```python
from build123d import *
from OCP.BRepFilletAPI import BRepFilletAPI_MakeFillet

# Parameters (mm, degrees)
SKETCH1_W                 = 28
SKETCH1_H                 = 28
BOSS_EXTRUDE1_DEPTH       = 66
SHELL1_T                  = -2
SHELL1_THICKNESS_2_FACE_W = 24
SHELL1_THICKNESS_2_FACE_H = 26
SHELL1_THICKNESS_2_DEPTH  = 1
SKETCH2_R                 = 2.5
SKETCH2_R_2               = 1.425
CUT_EXTRUDE4_DEPTH        = 2
SKETCH5_W                 = 14
SKETCH5_H                 = 5
CUT_EXTRUDE6_DEPTH        = 10
SKETCH6_R                 = 7
SKETCH6_R_2               = 1.1
CUT_EXTRUDE8_DEPTH        = 10
FILLET1_R                 = 0.5
BOSS_EXTRUDE2_START       = 8
BOSS_EXTRUDE2_DEPTH       = 32
SKETCH16_W                = 4
SKETCH16_H                = 2
BOSS_EXTRUDE9_DEPTH       = 1.5
SKETCH17_W                = 2.65
SKETCH17_H                = 2.3
CUT_EXTRUDE9_DEPTH        = 3
FILLET3_R                 = 1
FILLET3_R_2               = 0.5
CUT_EXTRUDE10_REACH       = 71.226
SKETCH18_W                = 14
SKETCH18_H                = 14


with BuildPart() as part:
    # Sketch1 → Boss-Extrude1 (new body)
    with BuildSketch(Plane.XY):
        Rectangle(SKETCH1_W, SKETCH1_H)
    extrude(amount=BOSS_EXTRUDE1_DEPTH)

    # Shell1
    shell1_openings = [part.faces().sort_by_distance(p)[0] for p in [
        (0, -14, 33),
    ]]
    offset(amount=SHELL1_T, openings=shell1_openings, kind=Kind.INTERSECTION)

    # Shell1 thickness 2 face (on inner face of the shell) → Shell1 thickness 2 (cut)
    with BuildSketch(Plane(origin=(0, -1, 64), x_dir=(1, 0, 0), z_dir=(0, 0, 1))):
        Rectangle(SHELL1_THICKNESS_2_FACE_W, SHELL1_THICKNESS_2_FACE_H)
    extrude(amount=SHELL1_THICKNESS_2_DEPTH, mode=Mode.SUBTRACT)

    # Sketch2 → Cut-Extrude4 (cut)
    with BuildSketch(Plane.XY):
        Circle(SKETCH2_R)
        with Locations((8.25, 0)):
            Circle(SKETCH2_R_2)
        with Locations((0, -8.25)):
            Circle(SKETCH2_R_2)
        with Locations((-8.25, 0)):
            Circle(SKETCH2_R_2)
        with Locations((0, 8.25)):
            Circle(SKETCH2_R_2)
    extrude(amount=CUT_EXTRUDE4_DEPTH, mode=Mode.SUBTRACT)

    # Sketch5 → Cut-Extrude6 (cut)
    with BuildSketch(Plane(origin=(0, 14, 0), x_dir=(1, 0, 0), z_dir=(0, 1, 0))):
        with Locations((0, -7.5)):
            Rectangle(SKETCH5_W, SKETCH5_H)
    extrude(amount=-CUT_EXTRUDE6_DEPTH, mode=Mode.SUBTRACT)

    # Sketch6 → Cut-Extrude8 (cut)
    with BuildSketch(Plane.XY.offset(66)):
        Circle(SKETCH6_R)
        with Locations((0, 9)):
            Circle(SKETCH6_R_2)
        with Locations((9, 0)):
            Circle(SKETCH6_R_2)
        with Locations((0, -9)):
            Circle(SKETCH6_R_2)
        with Locations((-9, 0)):
            Circle(SKETCH6_R_2)
    extrude(amount=-CUT_EXTRUDE8_DEPTH, mode=Mode.SUBTRACT)

    # Fillet1
    fillet1_edges = [part.edges().sort_by_distance(p)[0] for p in [
        (-7, 13, 5),
        (7, 13, 5),
        (7, 13, 10),
        (-7, 13, 10),
    ]]
    fillet(fillet1_edges, radius=FILLET1_R)

    # Sketch9 → Boss-Extrude2 (add)
    with BuildSketch(Plane.XY.offset(2).offset(BOSS_EXTRUDE2_START)):
        with BuildLine():
            ThreePointArc((6.82202316, 7.65), (9.353829093, 4.191465293), (10.25, 0))
            Line((10.25, 0), (12, 0))
            Line((12, 0), (12, 12))
            Line((12, 12), (-12, 12))
            Line((-12, 12), (-12, 0))
            Line((-12, 0), (-10.25, 0))
            ThreePointArc((-10.25, 0), (-9.353829093, 4.191465293), (-6.82202316, 7.65))
            ThreePointArc((-6.82202316, 7.65), (0, 10.25), (6.82202316, 7.65))
        make_face()
        with BuildLine():
            Line((-6.82202316, 7.65), (-1.292526595, 7.65))
            ThreePointArc((-1.292526595, 7.65), (-0.307225163, 9.641487585), (1.425, 8.25))
            ThreePointArc((1.425, 8.25), (1.391487585, 7.942774837), (1.292526595, 7.65))
            Line((1.292526595, 7.65), (6.82202316, 7.65))
            ThreePointArc((6.82202316, 7.65), (0, 10.25), (-6.82202316, 7.65))
        make_face()
        with BuildLine():
            Line((-1.292526595, 7.65), (0, 7.65))
            Line((0, 7.65), (1.292526595, 7.65))
            ThreePointArc((1.292526595, 7.65), (1.391487585, 7.942774837), (1.425, 8.25))
            ThreePointArc((1.425, 8.25), (-0.307225163, 9.641487585), (-1.292526595, 7.65))
        make_face()
    extrude(amount=BOSS_EXTRUDE2_DEPTH)

    # Sketch16 → Boss-Extrude9 (add)
    with BuildSketch(Plane.XZ.offset(14)):
        with Locations((-2, 1)):
            Rectangle(SKETCH16_W, SKETCH16_H)
        with Locations((2, 1)):
            Rectangle(SKETCH16_W, SKETCH16_H)
    extrude(amount=BOSS_EXTRUDE9_DEPTH)

    # Sketch17 → Cut-Extrude9 (cut)
    with BuildSketch(Plane.XY.offset(2)):
        with Locations((1.325, -12.85)):
            Rectangle(SKETCH17_W, SKETCH17_H)
        with Locations((-1.325, -12.85)):
            Rectangle(SKETCH17_W, SKETCH17_H)
    extrude(amount=-CUT_EXTRUDE9_DEPTH, mode=Mode.SUBTRACT)

    # Fillet3
    fillet3_edges_1 = [part.edges().sort_by_distance(p)[0] for p in [
        (-4, -15.5, 1),
        (4, -15.5, 1),
    ]]
    fillet3_edges_2 = [part.edges().sort_by_distance(p)[0] for p in [
        (4, -14, 1),
        (-4, -14, 1),
    ]]
    fillet3 = BRepFilletAPI_MakeFillet(part.part.solid().wrapped)
    for e in fillet3_edges_1:
        fillet3.Add(FILLET3_R - 0.0001, e.wrapped)
    for e in fillet3_edges_2:
        fillet3.Add(FILLET3_R_2 - 0.0001, e.wrapped)
    add(Compound.cast(fillet3.Shape()), mode=Mode.REPLACE)  # a hair under: the kernel refuses the full size

    # Sketch18 → Cut-Extrude10 (cut, up to next)
    with BuildSketch(Plane.XY.offset(66), mode=Mode.PRIVATE) as cut_extrude10_sk1:
        with Locations((0, -7)):
            Rectangle(SKETCH18_W, SKETCH18_H)
    cut_extrude10_tool1 = extrude(cut_extrude10_sk1.sketch, amount=-CUT_EXTRUDE10_REACH, mode=Mode.PRIVATE) & part.part
    add(cut_extrude10_tool1.solids().sort_by_distance((0, -7, 66))[0], mode=Mode.SUBTRACT)


solid = part.part
```
CAD build for the part. Positions are in the model's coordinates, mm. A direction names the side the tool comes from. Round coordinates to 2 decimals unless told otherwise and drop trailing zeros. Order: outer loops, then holes, each group sorted by start corner. A loop starts at its lowest first (then second) coordinate and runs counter-clockwise, first axis right, second up. Notation, with made-up numbers: (-38, 89) -> (-10, 89) arc R22 ccw to (-10, 102) -> close; hole circle Ø6 at (-4, 44.25). An arc over 180 degrees is marked (long way). One line per question, with ' | ' between items.
Q1. Slice it at A-A (x = 0). Give the number of separate pieces and of enclosed holes in the cut face, then the cut area to 3 significant figures.
Completed:
separate pieces: 7 | enclosed holes: 0 | area: 293 mm^2
Q2. Drop flat-ended pins along their axis: pin 1 (1.5 mm diameter, centred on x = 5, y = -6, fed in from +Z); pin 2 (10 mm diameter, centred on x = 10.5, z = 33.5, fed in from -Y); pin 3 (4 mm diameter, centred on x = 5.5, z = 33, fed in from -Y). Give the stop position or say it passes through.
Completed:
pin 1: stops at z = 2 | pin 2: stops at y = -14 | pin 3: stops at y = 6.99
Q3. Two-plate mould, pull along X, no slides. Class faces 5 (the flat face through (0, 9, 10)), 6 (the flat face through (-3, -1, 0)), 7 (the flat face through (-14, 0, 33)): released by +X, released by -X, zero draft, split by the parting line, or undercut.
Completed:
face 5: undercut | face 6: zero draft | face 7: released by -X
Q4. Slice it at C-C (x = -5.5). Write the cut outline in (y, z), then the cut area to 3 significant figures.
Completed:
outline: (-14, 0) -> (14, 0) -> (14, 5) -> (12, 5) -> (12, 2) -> (-14, 2) -> close; (4.33, 65) -> (12, 65) -> (12, 42) -> (7.65, 42) -> (7.65, 10) -> (14, 10) -> (14, 66) -> (4.33, 66) -> close | area: 321 mm^2
Q5. Which spindle directions (+Z, -Z, +X, -X, +Y, -Y) get a long thin tool onto all of the face, cutting with end or side? Do faces 1 (the flat face through (11, 0, 26)), 2 (the flat face through (2.65, -13, 1)), 3 (the flat face through (7, 13, 8)), 4 (the cylindrical face through (-9.674, 0.063, 0.986)). Say none if no direction does.
Completed:
face 1: -Y | face 2: +Z, -Z | face 3: +Y, -Y | face 4: -Z
Q6. Probe probe 1 along Z at (x, y) = (-9.25, 9); probe 2 along Y at (x, z) = (-8.25, 1) (3 decimals); probe 3 along X at (y, z) = (-8, 48). List the from-to ranges inside material, lowest first.
Completed:
probe 1: z = 0 to 2, 10 to 42, 65 to 66 | probe 2: y = -14 to -1.425, 1.425 to 14 | probe 3: x = -14 to -12, 12 to 14
Q7. Slice it at D-D (y = -4.75). Write the cut outline in (x, z).
Completed:
outline: (-14, 0) -> (14, 0) -> (14, 66) -> (7, 66) -> (7, 65) -> (12, 65) -> (12, 2) -> (-12, 2) -> (-12, 65) -> (-7, 65) -> (-7, 66) -> (-14, 66) -> close
Q8. Slice it at B-B (z = 51.5). Write the cut outline in (x, y), then the cut area to 3 significant figures.
Completed:
outline: (-14, -14) -> (-12, -14) -> (-12, 12) -> (12, 12) -> (12, -14) -> (14, -14) -> (14, 14) -> (-14, 14) -> close | area: 160 mm^2
